Check sheet for the modelled part. Datum: model origin and axes. Units: mm. A direction names the side the tool comes from. Give positions to 0.01 mm unless a question says otherwise; leave off trailing zeros. Write each loop counter-clockwise with the first axis right and the second up, starting at its lowest first coordinate (ties: lowest second). Pieces come first, ordered by that corner, then holes. Notation, with made-up numbers: (33, -1) -> (74, -1) arc R24 ccw to (74, 38) -> close; hole circle Ø4 at (52.25, 28.25). An arc over 180 degrees is marked (long way). Answer as a JSON object with one key per item and string values.
from build123d import *

# Parameters (mm, degrees)
ESTRUSIONE_ESTRUSIONE1_DEPTH = 30
ESTRUSIONE_ESTRUSIONE2_DEPTH = 7
FORO_10_0_10_1_D             = 10
FORO_10_0_10_1_CSINK_D       = 10.05
FORO_10_0_10_1_CSINK_ANGLE   = 90
FORO_4_0_4_1_D               = 4
FORO_4_0_4_1_CSINK_D         = 4.05
FORO_4_0_4_1_CSINK_ANGLE     = 90
SMUSSO1_SIZE                 = 5
RACCORDO1_R                  = 2
RACCORDO2_R                  = 6
RACCORDO3_R                  = 5
TAGLIO_ESTRUSIONE4_DEPTH     = 3
TAGLIO_ESTRUSIONE4_DRAFT     = 60


with BuildPart() as part:
    # Schizzo1 → Estrusione-Estrusione1 (new, symmetric)
    with BuildSketch(Plane.XY):
        Polygon((0, 44), (0, 0), (37, 0), (37, 4), (12, 4), (12, 44), align=None)
    extrude(amount=ESTRUSIONE_ESTRUSIONE1_DEPTH, both=True)

    # Schizzo3 → Estrusione-Estrusione2 (add)
    with BuildSketch(Plane(origin=(0, 4, 0), x_dir=(1, 0, 0), z_dir=(0, 1, 0))):
        Polygon((12, 30), (18, 30), (18, 4), (37, 4), (37, -4), (18, -4), (18, -30), (12, -30), align=None)
    extrude(amount=ESTRUSIONE_ESTRUSIONE2_DEPTH)

    # Foro Ø10.0 (10)-1 (through all)
    with Locations(Plane(origin=(12, 27.5, 0), x_dir=(0, 0, 1), z_dir=(1, 0, 0))):
        with Locations((0, 0)):
            CounterSinkHole(FORO_10_0_10_1_D / 2, FORO_10_0_10_1_CSINK_D / 2, counter_sink_angle=FORO_10_0_10_1_CSINK_ANGLE)

    # Foro Ø4.0 (4)-1 (through all)
    with Locations(Plane(origin=(15, 11, -24), x_dir=(1, 0, 0), z_dir=(0, 1, 0))):
        with Locations((0, 0), (16, -24), (0, -48)):
            CounterSinkHole(FORO_4_0_4_1_D / 2, FORO_4_0_4_1_CSINK_D / 2, counter_sink_angle=FORO_4_0_4_1_CSINK_ANGLE)

    # Smusso1
    smusso1_edges = [part.edges().sort_by_distance(p)[0] for p in [
        (37, 2, 30),
        (37, 2, -30),
    ]]
    chamfer(smusso1_edges, length=SMUSSO1_SIZE)

    # Raccordo1
    raccordo1_edges = [part.edges().sort_by_distance(p)[0] for p in [
        (18, 7.5, 30),
        (37, 7.5, 4),
        (37, 7.5, -4),
        (18, 7.5, -30),
    ]]
    fillet(raccordo1_edges, radius=RACCORDO1_R)

    # Raccordo2
    raccordo2_edges = [part.edges().sort_by_distance(p)[0] for p in [
        (18, 7.5, 4),
        (18, 7.5, -4),
    ]]
    fillet(raccordo2_edges, radius=RACCORDO2_R)

    # Raccordo3
    raccordo3_edges = [part.edges().sort_by_distance(p)[0] for p in [
        (6, 44, 30),
        (6, 44, -30),
    ]]
    fillet(raccordo3_edges, radius=RACCORDO3_R)


with BuildPart() as taglio_estrusione4_tool:
    # Schizzo2 → Taglio-Estrusione4 (with draft: the straight prism first)
    with BuildSketch(Plane(origin=(12, 0, 0), x_dir=(0, 0, -1), z_dir=(1, 0, 0))):
        with BuildLine():
            Line((-10, 42.375961669), (-10, 27.5))
            ThreePointArc((-10, 27.5), (0, 17.5), (10, 27.5))
            Line((10, 27.5), (10, 42.375961669))
            Line((10, 42.375961669), (10, 44))
            Line((10, 44), (-10, 44))
            Line((-10, 44), (-10, 42.375961669))
        make_face()
    extrude(amount=-TAGLIO_ESTRUSIONE4_DEPTH)
    # Taglio-Estrusione4: the draft: its side faces are tilted about the plane it starts from
    taglio_estrusione4_sides = [taglio_estrusione4_tool.faces().sort_by_distance(p)[0] for p in [
        (10.5, 35.75, 10),
        (10.5, 35.75, -10),
        (10.5, 44, 0),
        (10.5, 17.5, 0),
    ]]
    draft(taglio_estrusione4_sides, Plane(origin=(12, 0, 0), x_dir=(0, 0, -1), z_dir=(1, 0, 0)), TAGLIO_ESTRUSIONE4_DRAFT)


with BuildPart() as part_1:
    add(part.part)

    # Taglio-Estrusione4: cut by taglio_estrusione4_tool
    add(taglio_estrusione4_tool.part, mode=Mode.SUBTRACT)


solid = part_1.part
1. Sectioned sample at A-A, the plane z = 24. Enter the section's corners in (x, y) (3 decimals).
Determined:
{"outline": "(0, 0) -> (13, 0) -> (13, 10.975) -> (12.975, 11) -> (12, 11) -> (12, 44) -> (0, 44) -> close; (17, 0) -> (37, 0) -> (37, 4) -> (18, 4) -> (18, 11) -> (17.025, 11) -> (17, 10.975) -> close"}
2. Access from +Z, -Z, +X, -X, +Y, -Y to the whole of each face (thin tool, end or side, straight path). Record for faces 1 (the face through (9, 32, 4)), 2 (the face through (18, 7, -19)), 3 (the face through (27, 4, 16)).
Determined:
{"face 1": "+Y", "face 2": "-Z, +X, +Y", "face 3": "+Z, +X, +Y"}
3. Scan lines: L1, parallel to Z at x = 15, y = 2; L2, parallel to X at y = 8, z = 24; L3, parallel to Y at x = 5.75, z = 0. Record each from-to range of solid material in increasing order. Write a range as [from, to].
Determined:
{"L1": "[-30, -26], [-22, 22], [26, 30]", "L2": "[0, 13], [17, 18]", "L3": "[0, 22.5], [32.5, 44]"}
4. Sectioned sample at C-C, the plane y = 37.5. Enter the section's corners in (x, z), plus the area to 3 significant figures.
Determined:
{"outline": "(0, -30) -> (12, -30) -> (12, -10) -> (9, -15.2) -> (9, 15.2) -> (12, 10) -> (12, 30) -> (0, 30) -> close", "area": "644 mm^2"}
5. Sectioned sample at D-D, the plane x = 8. Enter the section's corners in (y, z).
Determined:
{"outline": "(0, -30) -> (39, -30) arc R5 ccw to (44, -25) -> (44, 25) arc R5 ccw to (39, 30) -> (0, 30) -> close; hole circle Ø10 at (27.5, 0)"}
6. Mould release check, pull along Z, two halves, no side actions. Record for faces 4 (the face through (4.44, 32.38, 1.08)), 5 (the face through (36.43, 7.55, -3.4)), 6 (the face through (0, 22, 0)): released by +Z, released by -Z, zero draft, split by the parting line, or undercut.
Determined:
{"face 4": "undercut", "face 5": "released by -Z", "face 6": "zero draft"}
7. Sectioned sample at B-B, the plane x = 31. Enter the section's corners in (y, z) (3 decimals).
Determined:
{"outline": "(0, -30) -> (4, -30) -> (4, -4) -> (11, -4) -> (11, -2.025) -> (10.975, -2) -> (0, -2) -> close; (0, 2) -> (10.975, 2) -> (11, 2.025) -> (11, 4) -> (4, 4) -> (4, 30) -> (0, 30) -> close"}
8. Go/stop test with flat-tipped pins: P1, Ø6, axis at y = 27.5, z = 0, coming from the +X side; P2, Ø8, axis at y = 27.5, z = 17.5, coming from the +X side; P3, Ø3.5, axis at y = 8, z = -16.5, coming from the +X side; P4, Ø2, axis at x = 29, y = 7, coming from the -Z side. Record where each tip stops, or that it passes through.
Determined:
{"P1": "through", "P2": "x = 12", "P3": "x = 18", "P4": "z = -4"}
